CAD build for the part. Positions are in the model's coordinates, mm. Face numbers are marked on the shaded views. A direction names the side the tool comes from. Round coordinates to 2 decimals unless told otherwise and drop trailing zeros. Loops run counter-clockwise (first coordinate to the right, second up) from the corner with the lowest first, then second, coordinate; pieces in that order, holes last. Notation, with made-up numbers: M 50,-30.75 L 63,-30.75 A23 cw 63,-19.75 Z; hole C 73,-22 d9. An arc over 180 degrees is marked long. One line per item, written item: value. Start each with the question number.
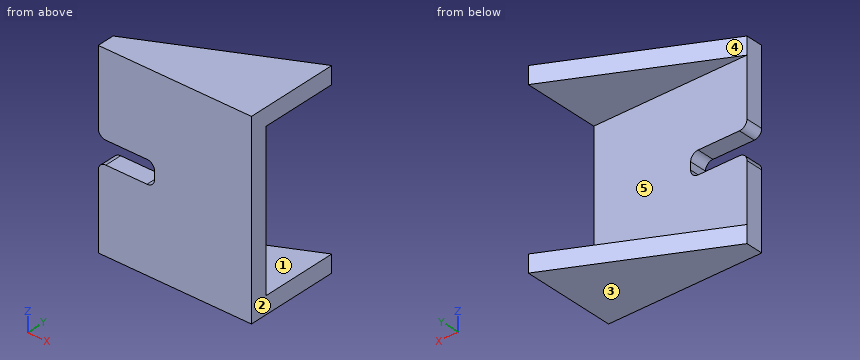
Autodesk Inventor part; units mm, degrees
ref_plane "YZ Plane" through (0, 0, 0) normal (1, 0, 0) x (0, 1, 0)
ref_plane "XZ Plane" through (0, 0, 0) normal (0, 1, 0) x (-1, 0, 0)
ref_plane "XY Plane" through (0, 0, 0) normal (0, 0, 1) x (1, 0, 0)
sketch "スケッチ1" plane through (0, 0, 0) normal (1, 0, 0) x (0, 1, 0)
  line L0 (-12.5, 12.5) -> (12.5, 12.5)
  line L1 (12.5, 12.5) -> (12.5, -12.5)
  line L2 (12.5, -12.5) -> (-12.5, -12.5)
  line L3 (-12.5, -12.5) -> (-12.5, 12.5)
  line L4 (-12.5, 12.5) -> (12.5, -12.5) construction
  line L5 (12.5, 12.5) -> (-12.5, -12.5) construction
  line L6 (10.2, 10.2) -> (-10.2, 10.2)
  line L7 (-10.2, 10.2) -> (-10.2, -10.2)
  line L8 (-10.2, -10.2) -> (10.2, -10.2)
  line L9 (10.2, -10.2) -> (10.2, 10.2)
  point P0 (0, 0)
  dimension "d0" = 25
  dimension "d1" = 25
  dimension "d2" = 2.3
extrude "押し出し1" add sketch "スケッチ1" along normal blind 25
sketch "スケッチ2" plane through (0, -12.5, 12.5) normal (0, 0, 1) x (1, 0, 0)
  line L0 (25, 25) -> (25, 0)
  line L1 (0, 12.5) -> (25, 12.5)
  line L2 (25, 12.5) -> (25, 25)
  line L3 (25, 25) -> (0, 25)
  line L4 (0, 25) -> (0, 12.5)
extrude "押し出し2" cut sketch "スケッチ2" against normal through all
sketch "スケッチ3" plane through (0, -12.5, 12.5) normal (0, 0, 1) x (1, 0, 0)
  line L0 (0, 0) -> (0, 12.5)
  line L1 (0, 0) -> (25, 12.5)
  line L2 (25, 12.5) -> (0, 12.5)
extrude "押し出し3" cut sketch "スケッチ3" against normal through all
sketch "スケッチ4" plane through (25, -10.2, 10.2) normal (0, 1, 0) x (1, 0, 0)
  line L0 (-25, -2.3) -> (0, -2.3)
  line L1 (-25, 22.7) -> (0, 22.7)
  line L2 (-25, -2.3) -> (-20.4, -2.3)
  line L3 (-20.4, -2.3) -> (-20.4, 22.7)
  line L4 (-20.4, 22.7) -> (-25, 22.7)
  line L5 (-25, 22.7) -> (-25, -2.3)
  line L6 (-20.4, 20.4) -> (-20.4, 0)
  point P0 (-25, 10.2)
extrude "押し出し4" cut sketch "スケッチ4" against normal blind 10
sketch "スケッチ5" plane through (25, -10.2, 10.2) normal (0, 1, 0) x (1, 0, 0)
  line L0 (-20.4, 8.7) -> (-12.9, 8.7)
  line L1 (-12.9, 8.7) -> (-12.9, 11.7)
  line L2 (-12.9, 11.7) -> (-20.4, 11.7)
  line L3 (-20.4, 11.7) -> (-20.4, 8.7)
  line L4 (-20.4, 20.4) -> (-20.4, 0)
  point P0 (-25, 10.2)
  point P1 (-20.4, 10.2)
  dimension "d11" = 3
  dimension "d12" = 7.5
extrude "押し出し5" cut sketch "スケッチ5" against normal blind 10
fillet "フィレット1" radius 1 4 edges at (4.6, -11.35, -1.5) (4.6, -11.35, 1.5) (12.1, -11.35, -1.5) (12.1, -11.35, 1.5)
equation "\"d1\" = d0"
properties part number "wire lead"
(1) Probe L1, parallel to Z at x = 8.75, y = -11; L2, parallel to Z at x = 9.75, y = -10; L3, parallel to Y at x = 10.25, z = -6.25. List the from-to ranges inside material, lowest first.
(2) Slice it at A-A, the plane y = -7.25. List the corners of the cut face in (x, z).
(3) Mould opens along Z. For the marked faces 3, 4 and 5 say: pulls with the +Z half, pulls with the -Z half, needs draft (parallel to the pull), parting line crosses it, or undercut.
(4) Slice it at B-B, the plane x = 11.5. List the corners of the cut face in (y, z).
(5) Slice it at D-D, the plane x = 18. List the corners of the cut face in (y, z).
(6) Flat gauge pin, fed straight in: P1, Ø3, axis at x = 11, z = -1.5, coming from the +Y side. Where does the tip first touch, or does it go through?
(7) Which spindle directions (+Z, -Z, +X, -X, +Y, -Y) get a long thin tool onto all of the face, cutting with end or side? Do the marked faces 1 and 2. Say none if no direction does.
(8) Slice it at C-C, the plane y = -2.75. List the corners of the cut face in (x, z), and give its area (3 significant figures).
Check result:
1. L1: z = -12.5 to -1.5, 1.5 to 12.5
1. L2: z = -12.5 to -10.2, 10.2 to 12.5
1. L3: y = -12.5 to -10.2
2. outline: M 10.5,-12.5 L 25,-12.5 L 25,-10.2 L 10.5,-10.2 Z; M 10.5,10.2 L 25,10.2 L 25,12.5 L 10.5,12.5 Z
3. face 3: pulls with the -Z half
3. face 4: needs draft
3. face 5: undercut
4. outline: M -12.5,-12.5 L -6.75,-12.5 L -6.75,-10.2 L -10.2,-10.2 L -10.2,-1.42 L -12.5,-1.42 Z; M -12.5,1.42 L -10.2,1.42 L -10.2,10.2 L -6.75,10.2 L -6.75,12.5 L -12.5,12.5 Z
5. outline: M -12.5,-12.5 L -3.5,-12.5 L -3.5,-10.2 L -10.2,-10.2 L -10.2,10.2 L -3.5,10.2 L -3.5,12.5 L -12.5,12.5 Z
6. P1: stops at y = -10.2
7. face 1: +X, -X, +Y
7. face 2: +Z, -Z, +X, +Y, -Y
8. outline: M 19.5,-12.5 L 25,-12.5 L 25,-10.2 L 19.5,-10.2 Z; M 19.5,10.2 L 25,10.2 L 25,12.5 L 19.5,12.5 Z
8. area: 25.3 mm^2
